from build123d import *

# Parameters (mm, degrees)
F0_R        = 24
F0_R_2      = 1.5
F1_DEPTH    = 3
F2_COUNT    = 5
F3_T1_DEPTH = 3
F4_R        = 1


# Not quite as in the source:
# - a fillet or chamfer that OpenCascade refuses, or shapes differently, is made with other operations: its cross-section is extruded or revolved along the edge and cut away or added


with BuildPart() as f1:
    # F0 (on Front) → F1 (new body)
    with BuildSketch(Plane.XZ):
        Circle(F0_R)
        with BuildLine():
            ThreePointArc((-1.4988309156, 18.9407894737), (0, 19), (1.4988309156, 18.9407894737))
            ThreePointArc((1.4988309156, 18.9407894737), (13.9548878067, 12.8942276349), (19, 0))
            ThreePointArc((19, 0), (-12.8942276349, -13.9548878067), (-1.4988309156, 18.9407894737))
        make_face(mode=Mode.SUBTRACT)
        with BuildLine():
            ThreePointArc((-1.9499920861, 4.0555555556), (-2.3953116303, -3.8095251927), (4.5, 0))
            ThreePointArc((4.5, 0), (3.8095251927, 2.3953116303), (1.9499920861, 4.0555555556))
            ThreePointArc((1.9499920861, 4.0555555556), (0, 4.5), (-1.9499920861, 4.0555555556))
        make_face()
        Circle(F0_R_2, mode=Mode.SUBTRACT)
        with BuildLine():
            ThreePointArc((-1.9499920861, 4.0555555556), (0, 4.5), (1.9499920861, 4.0555555556))
            Line((1.9499920861, 4.0555555556), (1.4988309156, 18.9407894737))
            ThreePointArc((1.4988309156, 18.9407894737), (0, 19), (-1.4988309156, 18.9407894737))
            Line((-1.4988309156, 18.9407894737), (-1.9499920861, 4.0555555556))
        make_face()
    extrude(amount=F1_DEPTH)

    # F2: F1 ×5 about axis
    f2_axis = Axis((0, 0, 0), (0, 1, 0))


with BuildPart() as f1_1:
    add(f1.part)
    for i in range(1, F2_COUNT):
        add(f1.part.rotate(f2_axis, i * 360 / F2_COUNT))

    # F3: fillet of radius 3 on 4 edges, made by hand

    # F3_s2 → F3_t1 (join)
    with BuildSketch(Plane.XZ):
        with BuildLine():
            ThreePointArc((-2.9413516087, 3.4056498225), (-2.1935950838, 4.3864419946), (-1.903629714, 5.5851968442))
            Line((-1.903629714, 5.5851968442), (-1.9499920861, 4.0555555556))
            ThreePointArc((-1.9499920861, 4.0555555556), (-2.467165408, 3.7633887454), (-2.9413516087, 3.4056498225))
        make_face()
        with BuildLine():
            ThreePointArc((2.3300378224, 3.8497952863), (3.4938960826, 3.4417180197), (4.7235839209, 3.5363801859))
            Line((4.7235839209, 3.5363801859), (3.2544818448, 3.1077882685))
            ThreePointArc((3.2544818448, 3.1077882685), (2.8167993507, 3.5093648169), (2.3300378224, 3.8497952863))
        make_face()
        with BuildLine():
            ThreePointArc((1.903629714, 5.5851968442), (2.1935950838, 4.3864419946), (2.9413516087, 3.4056498225))
            ThreePointArc((2.9413516087, 3.4056498225), (2.467165408, 3.7633887454), (1.9499920861, 4.0555555556))
            Line((1.9499920861, 4.0555555556), (1.903629714, 5.5851968442))
        make_face()
        with BuildLine():
            ThreePointArc((5.9000917861, -0.0845387023), (4.8496124019, -0.7307477774), (4.1478930895, -1.7449879421))
            ThreePointArc((4.1478930895, -1.7449879421), (4.3415914287, -1.1834626593), (4.4596432318, -0.6013170919))
            Line((4.4596432318, -0.6013170919), (5.9000917861, -0.0845387023))
        make_face()
    extrude(amount=F3_T1_DEPTH)

    # F4
    f4_edges = [f1_1.edges().sort_by_distance(p)[0] for p in [
        (-1.498831, -1.5, 18.940789),
        (17.550597, -1.5, 7.278499),
        (18.476925, -1.5, 4.427553),
        (1.498831, -1.5, 18.940789),
    ]]
    fillet(f4_edges, radius=F4_R)


solid = f1_1.part
Design review of the part built by this model. Coordinates are the model's own, in mm. Round coordinates to 2 decimals unless told otherwise and drop trailing zeros. Order: outer loops, then holes, each group sorted by start corner. A loop starts at its lowest first (then second) coordinate and runs counter-clockwise, first axis right, second up.
1) Consider section B-B (y = -1.1). Count the separate pieces of the cut face and the enclosed holes in it, plus the area to 3 significant figures.
The answers:
separate pieces: 1
enclosed holes: 6
area: 986 mm2
2) Consider section A-A (x = 0). State the section outline as (y, z) points, plus the area to 3 significant figures.
The answers:
outline: (-3, -24) - (0, -24) - (0, -19) - (-3, -19) - close; (-3, -4.5) - (0, -4.5) - (0, -1.5) - (-3, -1.5) - close; (-3, 1.5) - (0, 1.5) - (0, 24) - (-3, 24) - close
area: 91.5 mm2
3) Consider section C-C (z = -18). State the section outline as (x, y) points.
The answers:
outline: (-15.87, -3) - (-6.08, -3) - (-6.08, 0) - (-15.87, 0) - close; (6.08, -3) - (15.87, -3) - (15.87, 0) - (6.08, 0) - close
4) Consider section D-D (z = 10.5). State the section outline as (x, y) points, plus the area to 3 significant figures.
The answers:
outline: (-21.58, -3) - (-15.84, -3) - (-15.84, 0) - (-21.58, 0) - close; (-1.75, -3) - (1.75, -3) - (1.75, 0) - (-1.75, 0) - close; (15.84, -3) - (21.58, -3) - (21.58, 0) - (15.84, 0) - close
area: 45.0 mm2
5) For L1, parallel to Z at x = 7, y = -1.7; L2, parallel to Z at x = -15.5, y = -2.8; L3, parallel to X at y = -0.4, z = 9, list the stretches that pass through material, from the lowest coordinate up.
The answers:
L1: z = -22.96 to -17.66, -12.43 to -6.6, 0.31 to 4.2, 17.66 to 22.96
L2: z = -18.32 to -10.99, 3.36 to 6.68, 10.99 to 18.32
L3: x = -22.25 to -16.73, -1.8 to 1.8, 16.73 to 22.25
